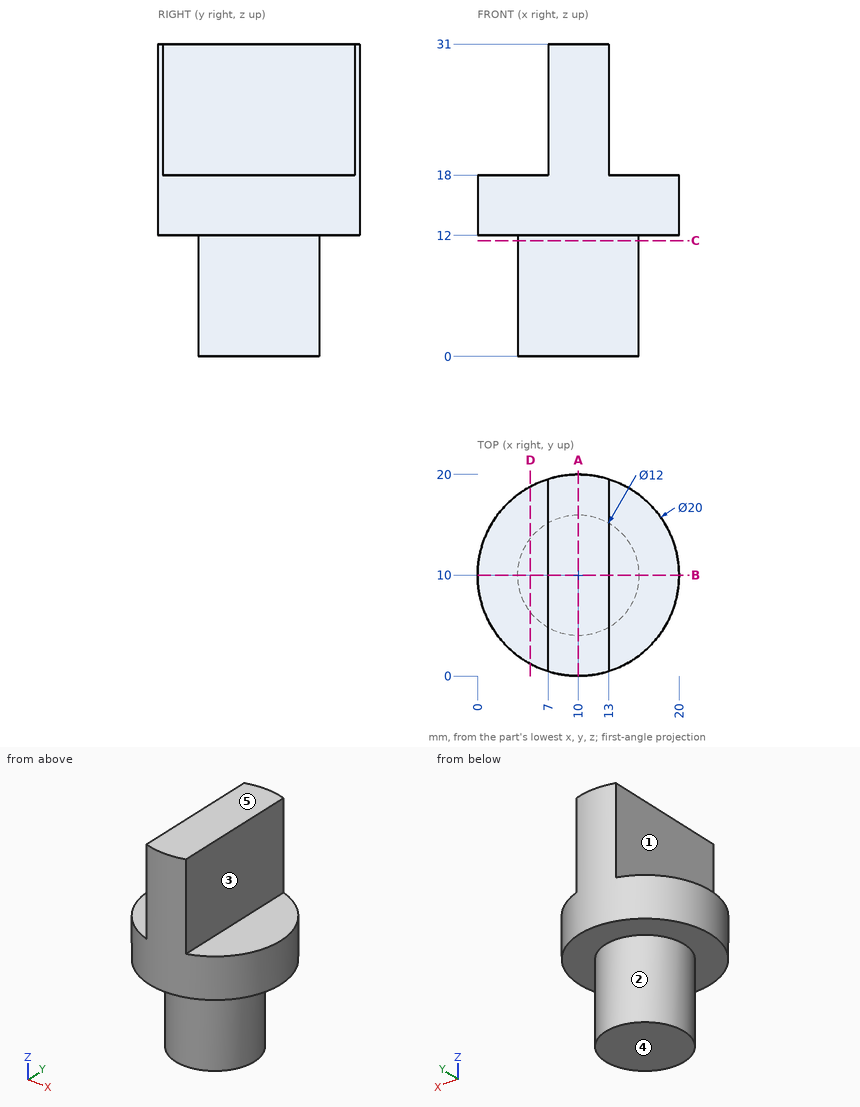
Check sheet for the drawn part. Datum: minimum x, y, z corner. Units: mm. A direction names the side the tool comes from. Round coordinates to 2 decimals unless told otherwise and drop trailing zeros. Loops run counter-clockwise (first coordinate to the right, second up) from the corner with the lowest first, then second, coordinate; pieces in that order, holes last. Notation, with made-up numbers: (34, 72) - (40, 72) arc R18 cw to (40, 76) - close; hole circle Ø10 at (75, 11). An arc over 180 degrees is marked (long way). Write item = value, one per line. Start each with the question number.
1. Section check B-B on y = 10. Enter the section's corners in (x, z).
2. Section check D-D on x = 5.25. Enter the section's corners in (y, z), then the cut area to 3 significant figures.
3. Set-up check for the marked faces 1, 2, 3, 4 and 5: record each of +Z, -Z, +X, -X, +Y, -Y from which the full face is reachable in a straight line by a thin tool's end or side.
4. Thickness scan on line 1 (X direction, y = 2.25, z = 23); line 2 (Z direction, x = 16.75, y = 13.5); line 3 (Z direction, x = 5.5, y = 10). Record the ranges inside material, lowest first.
5. Section check C-C on z = 11.5. Enter the section's corners in (x, y), then the cut area to 3 significant figures.
6. Depth check by flat-ended pin: pin 1 (12 mm diameter, centred on y = 2.5, z = 13.5, fed in from -X); pin 2 (8 mm diameter, centred on y = 17, z = 8.5, fed in from -X); pin 3 (4 mm diameter, centred on y = 8.5, z = 7.5, fed in from -X). Enter the tip coordinate at first touch or a pass-through.
7. Section check A-A on x = 10. Enter the section's corners in (y, z), then the cut area to 3 significant figures.
Working result:
q1.outline = (0, 12) - (4, 12) - (4, 0) - (16, 0) - (16, 12) - (20, 12) - (20, 18) - (13, 18) - (13, 31) - (7, 31) - (7, 18) - (0, 18) - close
q2.outline = (1.2, 12) - (6.33, 12) - (6.33, 0) - (13.67, 0) - (13.67, 12) - (18.8, 12) - (18.8, 18) - (1.2, 18) - close
q2.area = 194 mm^2
q3.face_1 = +Z, -X, +Y, -Y
q3.face_2 = -Z
q3.face_3 = +Z, +X, +Y, -Y
q3.face_4 = -Z, +X, -X, +Y, -Y
q3.face_5 = +Z, +X, -X, +Y, -Y
q4.line_1 = 7 to 13
q4.line_2 = 12 to 18
q4.line_3 = 0 to 18
q5.outline = circle Ø12 at (10, 10)
q5.area = 113 mm^2
q6.pin_1 = 0.11
q6.pin_2 = 1.38
q6.pin_3 = 4
q7.outline = (0, 12) - (4, 12) - (4, 0) - (16, 0) - (16, 12) - (20, 12) - (20, 31) - (0, 31) - close
q7.area = 524 mm^2
